Input: part model. Units: mm. Frame: model coordinates. Face numbers are marked on the shaded views. A direction names the side the tool comes from. Round coordinates to 2 decimals unless told otherwise and drop trailing zeros. Loops run counter-clockwise (first coordinate to the right, second up) from the corner with the lowest first, then second, coordinate; pieces in that order, holes last. Notation, with made-up numbers: (-28, 52) - (-20, 52) arc R18 ccw to (-20, 68) - close; hole circle Ø10 at (80.5, -28). An arc over 180 degrees is marked (long way). Write each question's results on one line, items separated by ' | '.
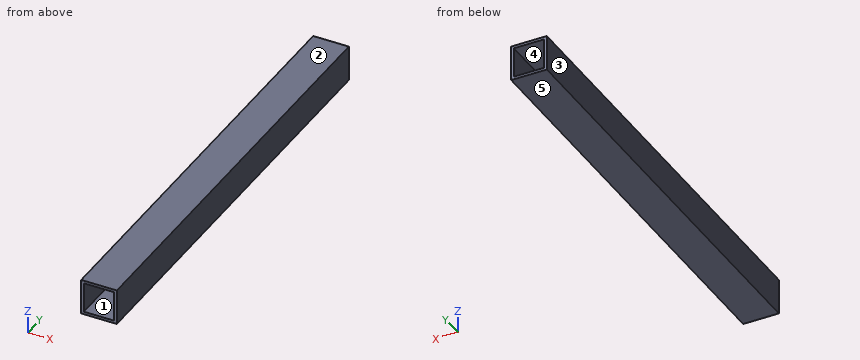
Autodesk Inventor part; units mm, degrees
ref_plane "YZ Plane" through (0, 0, 0) normal (1, 0, 0) x (0, 1, 0)
ref_plane "XZ Plane" through (0, 0, 0) normal (0, 1, 0) x (-1, 0, 0)
ref_plane "XY Plane" through (0, 0, 0) normal (0, 0, 1) x (1, 0, 0)
sketch "Sketch1" plane through (0, 0, 0) normal (0, 1, 0) x (-1, 0, 0)
  line L0 (-20, 20) -> (20, 20)
  line L1 (20, 20) -> (20, -20)
  line L2 (20, -20) -> (-20, -20)
  line L3 (-20, -20) -> (-20, 20)
  line L4 (-20, 20) -> (20, -20) construction
  line L5 (20, 20) -> (-20, -20) construction
  line L6 (-17, 17) -> (17, 17)
  line L7 (17, 17) -> (17, -17)
  line L8 (17, -17) -> (-17, -17)
  line L9 (-17, -17) -> (-17, 17)
  line L10 (-17, 17) -> (17, -17) construction
  line L11 (17, 17) -> (-17, -17) construction
  point P0 (0, 0)
  dimension "d0" = 40
  dimension "d1" = 40
  dimension "d2" = 34
  dimension "d3" = 34
  dimension "d4" = 3
extrude "Extrusion1" add sketch "Sketch1" along normal blind 490
properties part number "Tube 49 cm"
1. Mould query, pull axis X, two halves, no side actions, for the marked faces 3, 4 and 5. Classes: pulls with the +X half, pulls with the -X half, needs draft (parallel to the pull), parting line crosses it, or undercut.
Answer:
face 3: pulls with the -X half | face 4: undercut | face 5: needs draft
2. Set-up query: the marked faces 1 and 2. Return all of +Z, -Z, +X, -X, +Y, -Y with unobstructed straight access to the full face (end or side cutting, diameter ignored); none if empty.
Answer:
face 1: +Y, -Y | face 2: +Z, +X, -X, +Y, -Y
3. Section query C-C, the plane y = 241. Output: boundary loops of the cut face in (x, z), plus the area to 3 significant figures.
Answer:
outline: (-20, -20) - (20, -20) - (20, 20) - (-20, 20) - close; hole (-17, -17) - (17, -17) - (17, 17) - (-17, 17) - close | area: 444 mm^2
4. Section query A-A, the plane z = -6. Output: boundary loops of the cut face in (x, y), plus the area to 3 significant figures.
Answer:
outline: (-20, 0) - (-17, 0) - (-17, 490) - (-20, 490) - close; (17, 0) - (20, 0) - (20, 490) - (17, 490) - close | area: 2,940 mm^2
5. Section query B-B, the plane x = 0. Output: boundary loops of the cut face in (y, z).
Answer:
outline: (0, -20) - (490, -20) - (490, -17) - (0, -17) - close; (0, 17) - (490, 17) - (490, 20) - (0, 20) - close
6. Line query: line 1 (Z direction, x = 8.5, y = 466.5). Output: solid intervals per line, ascending. Write a range as [from, to].
Answer:
line 1: [-20, -17], [17, 20]
